Autodesk Inventor part; units mm, degrees
ref_plane "YZ Plane" through (0, 0, 0) normal (1, 0, 0) x (0, 1, 0)
ref_plane "XZ Plane" through (0, 0, 0) normal (0, 1, 0) x (-1, 0, 0)
ref_plane "XY Plane" through (0, 0, 0) normal (0, 0, 1) x (1, 0, 0)
sketch "Sketch1" plane through (0, 0, 0) normal (0, 0, 1) x (1, 0, 0)
  line L0 (-80, 105) -> (80, 105)
  line L1 (80, 105) -> (80, 5)
  line L2 (80, 5) -> (50, 5)
  line L3 (50, 5) -> (50, 0)
  line L4 (-50, 0) -> (-50, 5)
  line L5 (-50, 5) -> (-80, 5)
  line L6 (-80, 105) -> (-80, 5)
  line L7 (50, 0) -> (12.5, 0)
  line L8 (12.5, 0) -> (12.5, 5)
  line L9 (12.5, 5) -> (-12.5, 5)
  line L10 (-12.5, 5) -> (-12.5, 0)
  line L11 (-12.5, 0) -> (-50, 0)
  point P0 (0, 0)
  point P1 (0, 105)
  point P2 (0, 0)
  point P3 (0, 5)
  dimension "d0" = 5
  dimension "d1" = 100
  dimension "d2" = 160
  dimension "d3" = 100
  dimension "d22" = 5
  dimension "d23" = 25
  dimension "d24" = 5
  dimension "d25" = 30
extrude "Extrusion1" add sketch "Sketch1" along normal blind 5
sketch "Sketch3" plane through (0, 0, 0) normal (0, 0, -1) x (-1, 0, 0)
  line L0 (60, 13.5) -> (-60, 13.5) construction
  line L1 (-60, 13.5) -> (-60, 93.5) construction
  line L2 (-60, 93.5) -> (60, 93.5) construction
  line L3 (60, 93.5) -> (60, 13.5) construction
  line L4 (60, 13.5) -> (-60, 93.5) construction
  line L5 (-60, 13.5) -> (60, 93.5) construction
  line L6 (80, 5) -> (50, 5)
  point P0 (0, 0)
  point P1 (60, 93.5)
  point P2 (0, 53.5)
  point P3 (0, 93.5)
  dimension "d32" = 120
  dimension "d33" = 8.5
  dimension "d34" = 80
hole "Hole1" at (60, 93.5, 0) at (-60, 93.5, 0) at (60, 13.5, 0) at (-60, 13.5, 0) direction (0, 0, 1) diameter 3.4 depth 8 tip angle 118 countersink diameter 6.3 countersink angle 90
fillet "Fillet1" radius 4 2 edges at (80, 105, 2.5) (-80, 105, 2.5)
sketch "Sketch5" plane through (0, 0, 0) normal (0, 0, -1) x (-1, 0, 0)
  line L0 (-2.25, 5) -> (-2.25, 10)
  line L1 (-2.25, 10) -> (-3.5, 10)
  line L2 (-3.5, 10) -> (-3.5, 13.2)
  line L3 (-3.5, 13.2) -> (3.5, 13.2)
  line L4 (3.5, 13.2) -> (3.5, 10)
  line L5 (3.5, 10) -> (2.25, 10)
  line L6 (2.25, 10) -> (2.25, 5)
  line L7 (-12.5, 5) -> (12.5, 5)
  line L8 (-2.25, 5) -> (2.25, 5)
  point P0 (0, 0)
  point P1 (0, 13.2)
  point P2 (0, 5)
  point P3 (0, 5)
  dimension "d26" = 7
  dimension "d27" = 3.2
  dimension "d28" = 5
  dimension "d29" = 4.5
extrude "Extrusion3" cut sketch "Sketch5" against normal blind 5
equation "\"d25\" = -0.5 * d1 + 0.5 * d2"
properties part number "LogicHolder" material "Polycarbonate, Clear"
Geometry check sheet. Reference: the model listing, model coordinates, mm. A direction names the side the tool comes from. Coordinates: 2 decimals unless noted, no trailing zeros. Order: outer loops, then holes, each group sorted by start corner. A loop starts at its lowest first (then second) coordinate and runs counter-clockwise, first axis right, second up.
Item 1: Section check A-A (x = -60). Enter the section's corners in (y, z), plus the area to 3 significant figures.
Item 2: Mould release check, pull along Y, two halves, no side actions. Record for faces 6 (the flat face through (32, 0, 2)), 7 (the cylindrical face through (-61.433, 14.414, 3.25)), 8 (the flat face through (-80, 54, 2)), 9 (the flat face through (0, 13.2, 2)): released by +Y, released by -Y, zero draft, split by the parting line, or undercut.
Item 3: Tool access check on faces 1 (the flat face through (-3.5, 12, 2)), 2 (the flat face through (50, 3, 2)), 3 (the flat face through (-65, 5, 2)), 4 (the flat face through (-2.25, 8, 2)), 5 (the flat face through (80, 54, 2)). Record the directions out of +Z, -Z, +X, -X, +Y, -Y that give a thin tool (end or side, any length) a straight path to the whole face; none if there is none.
Item 4: Depth check by flat-ended pin: pin 1 (2.5 mm diameter, centred on y = 3.5, z = 2.5, fed in from +X); pin 2 (4.5 mm diameter, centred on x = -60, y = 93.5, fed in from -Z); pin 3 (2.5 mm diameter, centred on x = -71.5, z = 2, fed in from -Y). Enter the tip coordinate at first touch or a pass-through.
Item 5: Section check B-B (y = 93.5). Enter the section's corners in (x, z).
Item 6: Scan lines: line 1 along Y through (x, z) = (-60, 2.7); line 2 along X through (y, z) = (93.5, 3.5); line 3 along X through (y, z) = (6.5, 4.1). Record each from-to range of solid material in increasing order.
Check sheet entries:
1. outline: (5, 0) - (10.35, 0) - (11.8, 1.45) - (11.8, 5) - (5, 5) - close; (15.2, 1.45) - (16.65, 0) - (90.35, 0) - (91.8, 1.45) - (91.8, 5) - (15.2, 5) - close; (95.2, 1.45) - (96.65, 0) - (105, 0) - (105, 5) - (95.2, 5) - close
1. area: 462 mm2
2. face 6: released by -Y
2. face 7: undercut
2. face 8: zero draft
2. face 9: undercut
3. face 1: +Z, -Z
3. face 2: +Z, -Z, +X, -Y
3. face 3: +Z, -Z, -X, -Y
3. face 4: +Z, -Z, -Y
3. face 5: +Z, -Z, +X, +Y, -Y
4. pin 1: stops at x = 50
4. pin 2: stops at z = 0.9
4. pin 3: stops at y = 5
5. outline: (-80, 0) - (-63.15, 0) - (-61.7, 1.45) - (-61.7, 5) - (-80, 5) - close; (-58.3, 1.45) - (-56.85, 0) - (56.85, 0) - (58.3, 1.45) - (58.3, 5) - (-58.3, 5) - close; (61.7, 1.45) - (63.15, 0) - (80, 0) - (80, 5) - (61.7, 5) - close
6. line 1: y = 5 to 11.8, 15.2 to 91.8, 95.2 to 105
6. line 2: x = -80 to -61.7, -58.3 to 58.3, 61.7 to 80
6. line 3: x = -80 to -2.25, 2.25 to 80
